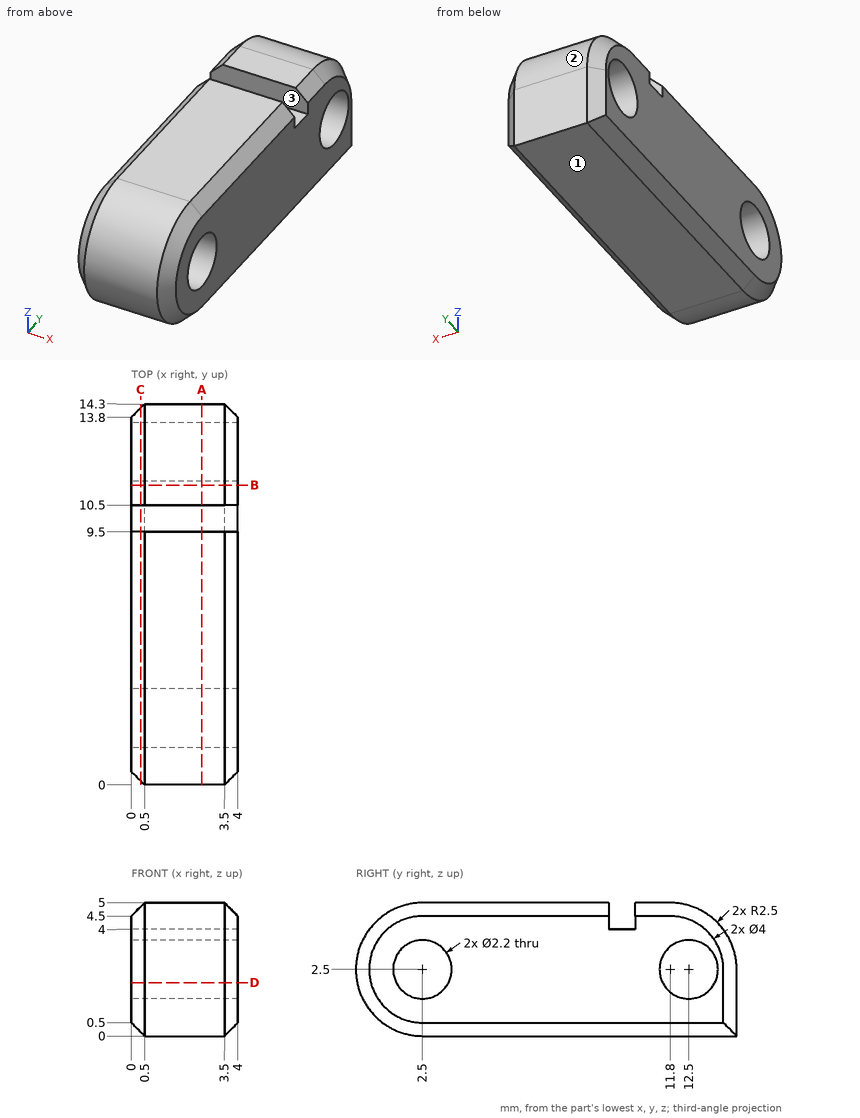
Geometry check sheet. Reference: drawing and pictorial views, mm from the part's lowest x, y, z. Coordinates: 2 decimals unless noted, no trailing zeros. Write each loop counter-clockwise with the first axis right and the second up, starting at its lowest first coordinate (ties: lowest second). Pieces come first, ordered by that corner, then holes.
Item 1: Cross-section at C-C on x = 0.35. Record the boundary of the cut face in (y, z).
Numbers:
outline: (2.5, 0.15) - (14.15, 0.15) - (14.15, 2.5) arc R2.35 ccw to (11.8, 4.85) - (10.5, 4.85) - (10.5, 4) - (9.5, 4) - (9.5, 4.85) - (2.5, 4.85) arc R2.35 ccw to start; hole circle Ø2.2 at (2.5, 2.5); hole circle Ø2.2 at (12.5, 2.5)
Item 2: Scan lines: probe 1 along Z at (x, y) = (2.85, 2.5); probe 2 along Y at (x, z) = (1.7, 3); probe 3 along Y at (x, z) = (1.6, 1.65). Record each from-to range of solid material in increasing order.
Numbers:
probe 1: z = 0 to 1.4, 3.6 to 5
probe 2: y = 0.05 to 1.52, 3.48 to 11.52, 13.48 to 14.25
probe 3: y = 0.15 to 1.8, 3.2 to 11.8, 13.2 to 14.3
Item 3: Cross-section at B-B on y = 11.25. Record the boundary of the cut face in (x, z).
Numbers:
outline: (0, 0.5) - (0.5, 0) - (3.5, 0) - (4, 0.5) - (4, 4.5) - (3.5, 5) - (0.5, 5) - (0, 4.5) - close
Item 4: Depth check by flat-ended pin: pin 1 Ø2 at (x, z) = (3, 4) entering from +Y; pin 2 Ø0.5 at (x, z) = (2, 4.5) entering from -Y; pin 3 Ø2 at (x, z) = (2.5, 1) entering from -Y. Enter the tip coordinate at first touch or a pass-through.
Numbers:
pin 1: stops at y = 14.25
pin 2: stops at y = 0.71
pin 3: stops at y = 0.05
Item 5: Mould release check, pull along Y, two halves, no side actions. Record for the marked faces 1, 2 and 3: released by +Y, released by -Y, zero draft, split by the parting line, or undercut.
Numbers:
face 1: zero draft
face 2: released by +Y
face 3: undercut
Item 6: Cross-section at A-A on x = 2.65. Record the boundary of the cut face in (y, z).
Numbers:
outline: (2.5, 0) - (14.3, 0) - (14.3, 2.5) arc R2.5 ccw to (11.8, 5) - (10.5, 5) - (10.5, 4) - (9.5, 4) - (9.5, 5) - (2.5, 5) arc R2.5 ccw to start; hole circle Ø2.2 at (2.5, 2.5); hole circle Ø2.2 at (12.5, 2.5)
Item 7: Cross-section at D-D on z = 2. Count the separate pieces of the cut face and the enclosed holes in it, then the cut area to 3 significant figures.
Numbers:
separate pieces: 3
enclosed holes: 0
area: 40.8 mm2
